Read the model definition and answer for the solid it produces. Units are mm, in the model's axes. Face numbers are marked on the shaded views. A direction names the side the tool comes from. Coordinates: 2 decimals unless noted, no trailing zeros. Loops run counter-clockwise (first coordinate to the right, second up) from the corner with the lowest first, then second, coordinate; pieces in that order, holes last. Notation, with made-up numbers: (-38.5, 56) -> (18.5, 56) arc R19 cw to (18.5, 78) -> close; hole circle Ø11 at (-20.5, 62.25). An arc over 180 degrees is marked (long way). Answer as a JSON object with one key per item and string values. Group by question number.
Q1. Each of these flat-tipped pins is pushed along its axis until it touches: P1, Ø1.5, axis at x = 15, z = 15, coming from the -Y side; P2, Ø5.5, axis at x = 20.5, z = 13, coming from the +Y side; P3, Ø6, axis at y = -4, z = 15, coming from the +X side. Where does it stop, or does it pass through?
Q2. The part is cut by section D-D on x = 0. Write down the section's boundary in (y, z) (3 decimals), and give its area (3 significant figures).
Q3. Determine the mould class of the marked faces 4, 5 and 6 for opening direction X: released by +X, released by -X, zero draft, split by the parting line, or undercut.
Q4. The part is cut by section C-C on z = 17.25. Write down the section's boundary in (x, y) (3 decimals).
Q5. Straight lines are drawn through the part: line 1 along Y through (x, z) = (0.5, 3.75); line 2 along Z through (x, y) = (25.4, -1.4); line 3 along X through (y, z) = (-8.5, 2.5). For each, find the intervals that lie inside material, in ascending order. Write a range as [from, to].
Q6. The part is cut by section A-A on x = 25.4. Write down the section's boundary in (y, z), and give its area (3 significant figures).
Q7. The part is cut by section B-B on y = 0. Write down the section's boundary in (x, z) (3 decimals).
Q8. For the marked faces 1, 2 and 3, determine the directions among +Z, -Z, +X, -X, +Y, -Y from which every point of the face is accessible in a straight line to the end or side of a thin tool.
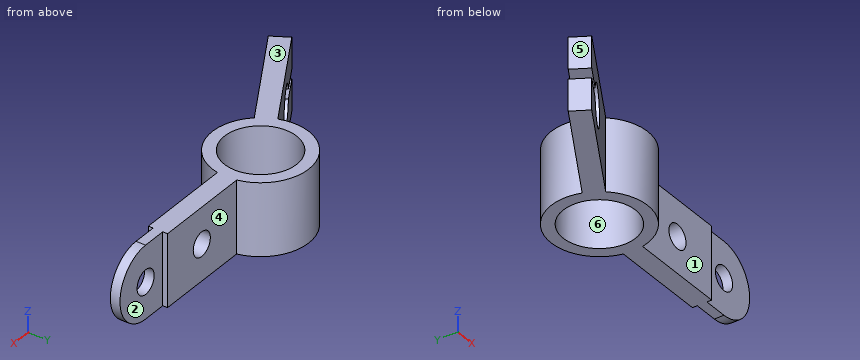
Autodesk Inventor part; units mm, degrees
ref_plane "YZ Plane" through (0, 0, 0) normal (1, 0, 0) x (0, 1, 0)
ref_plane "XZ Plane" through (0, 0, 0) normal (0, 1, 0) x (-1, 0, 0)
ref_plane "XY Plane" through (0, 0, 0) normal (0, 0, 1) x (1, 0, 0)
sketch "Boceto1" plane through (0, 0, 0) normal (0, 0, 1) x (1, 0, 0)
  circle A0 centre (0, 0) radius 9.525
  line L0 (12.4434, -2.54) -> (38.1, -2.54)
  line L1 (38.1, -2.54) -> (38.1, 2.54)
  line L2 (38.1, 2.54) -> (12.4434, 2.54)
  line L3 (12.7, 0) -> (9.5196, 0.3221) construction
  line L4 (9.5196, -0.3221) -> (12.7, 0) construction
  line L5 (-9.5063, -8.4214) -> (-37.2364, -24.4314)
  line L6 (-37.2364, -24.4314) -> (-39.7764, -20.032)
  line L7 (-39.7764, -20.032) -> (-12.0463, -4.022)
  line L8 (0.4725, -1.9521) -> (-1.0609, -2.54) construction
  arc A1 (12.4434, 2.54) -> (-12.0463, -4.022) centre (0, 0) ccw
  arc A2 (-9.5063, -8.4214) -> (12.4434, -2.54) centre (0, 0) ccw
  line L9 (38.1, -1.27) -> (44.45, -1.27)
  line L10 (44.45, -1.27) -> (44.45, 1.27)
  line L11 (44.45, 1.27) -> (38.1, 1.27)
  point P0 (-23.3714, -16.4264)
  point P1 (-38.5064, -22.2317)
  point P2 (41.275, -1.27)
  point P3 (41.275, 1.27)
  dimension "d0" = 19.05
  dimension "d3" = 5.08
  dimension "d4" = 2.54
  dimension "d7" = 5.08
  dimension "d8" = 38.5064
  dimension "d9" = 2.54
  dimension "d10" = 44.4634
  dimension "d11" = 3.175
  dimension "d12" = 3.175
  dimension "d13" = 38.1
  dimension "d14" = 6.35
  dimension "d16" = 2.54
  dimension "d17" = 1.27
extrude "Extrusión1" add sketch "Boceto1" along normal blind 19.05
sketch "Boceto2" plane through (38.1, 1.27, 0) normal (0, 1, 0) x (1, 0, 0)
  line L0 (6.35, 0) -> (0, 0)
  line L1 (6.35, -19.05) -> (0, -19.05)
  line L2 (6.35, 0) -> (6.35, -19.05)
  arc A0 (6.35, -19.05) -> (6.35, 0) centre (6.35, -9.525) ccw
  point P0 (-38.1, 0)
extrude "Extrusión2" add sketch "Boceto2" against normal blind 2.54
sketch "Boceto3" plane through (38.1, 1.27, 19.05) normal (0, 1, 0) x (1, 0, 0)
  line L0 (0, 19.05) -> (0, 0)
  line L1 (0, 19.05) -> (0, 9.525)
  line L2 (0, 19.05) -> (6.35, 19.05)
  line L3 (0, 0) -> (6.35, 0)
  line L4 (6.35, 19.05) -> (6.35, 0)
  line L5 (6.35, 0) -> (6.35, 9.525)
  circle A0 centre (6.35, 9.525) radius 3.175
  point P0 (-38.1, 19.05)
  dimension "d22" = 6.35
extrude "Extrusión3" cut sketch "Boceto3" against normal blind 2.54 contours A0 L4 | L4 A0
sketch "Boceto4" plane through (12.4434, 2.54, 0) normal (0, 1, 0) x (1, 0, 0)
  line L0 (25.7224, -0.5661) -> (25.7224, -18.5033)
  line L1 (25.7224, -18.5033) -> (25.6566, -9.525)
  line L2 (25.6566, 0) -> (25.6566, -19.05)
  line L3 (25.6566, -9.525) -> (12.9566, -9.525)
  circle A0 centre (12.9566, -9.525) radius 3.175
  point P0 (-12.4434, 0)
  dimension "d25" = 12.7
  dimension "d26" = 6.35
extrude "Extrusión4" cut sketch "Boceto4" against normal blind 5.08
sketch "Boceto5" plane through (-39.7764, -20.032, 19.05) normal (-0.5, 0.866, 0) x (0.866, 0.5, 0)
  line L0 (0, 19.05) -> (0, 0)
  line L1 (0, 0) -> (0, 19.05)
  line L2 (0, 19.05) -> (0, 9.525)
  line L3 (0, 9.525) -> (12.7, 9.525)
  circle A0 centre (12.7, 9.525) radius 5.08
  line L4 (7.7813, 8.255) -> (0, 8.255)
  line L5 (0, 8.255) -> (0, 10.795)
  line L6 (0, 10.795) -> (7.7813, 10.795)
  point P0 (44.4634, 19.05)
  point P1 (6.35, 9.525)
  point P2 (0, 10.795)
  point P3 (0, 8.255)
  dimension "d29" = 12.7
  dimension "d30" = 10.16
  dimension "d31" = 1.27
  dimension "d32" = 1.27
extrude "Extrusión5" cut sketch "Boceto5" against normal blind 5.08
properties part number "Pieza1-Tarea1"
Final values:
{
 "1": {"P1": "stops at y = -2.54", "P2": "stops at y = 2.54", "P3": "stops at x = 52.98"},
 "2": {"outline": "(-12.7, 0) -> (-9.525, 0) -> (-9.525, 19.05) -> (-12.7, 19.05) -> close; (9.525, 0) -> (12.7, 0) -> (12.7, 19.05) -> (9.525, 19.05) -> close", "area": "121 mm2"},
 "3": {"face 4": "zero draft", "face 5": "released by -X", "face 6": "undercut"},
 "4": {"outline": "(-39.776, -20.032) -> (-37.236, -24.431) -> (-9.506, -8.421) arc R12.7 ccw to (12.443, -2.54) -> (38.1, -2.54) -> (38.1, -1.27) -> (50.022, -1.27) -> (50.022, 1.27) -> (38.1, 1.27) -> (38.1, 2.54) -> (12.443, 2.54) arc R12.7 ccw (long way) to (-12.046, -4.022) -> close; hole circle Ø19.05 at (0, 0)"},
 "5": {"line 1": "y = [-12.69, -9.51], [9.51, 12.69]", "line 2": "z = [0, 6.35], [12.7, 19.05]", "line 3": "x = [-19.8, -9.64], [-9.44, -4.3], [4.3, 9.44]"},
 "6": {"outline": "(-2.54, 0) -> (2.54, 0) -> (2.54, 6.35) -> (-2.54, 6.35) -> close; (-2.54, 12.7) -> (2.54, 12.7) -> (2.54, 19.05) -> (-2.54, 19.05) -> close", "area": "64.5 mm2"},
 "7": {"outline": "(-12.7, 0) -> (-9.525, 0) -> (-9.525, 19.05) -> (-12.7, 19.05) -> close; (9.525, 0) -> (44.45, 0) arc R9.525 ccw to (44.45, 19.05) -> (9.525, 19.05) -> close; hole circle Ø6.35 at (25.4, 9.525); hole circle Ø6.35 at (44.45, 9.525)"},
 "8": {"face 1": "+Z, -Z, +X, -Y", "face 2": "+Z, -Z, +X, +Y", "face 3": "+Z, +X, -X, +Y, -Y"}
}
